The model under review builds one solid part; all positions refer to its coordinate system, in mm. Face numbers are marked on the shaded views. Coordinates: 2 decimals unless noted, no trailing zeros. Write each loop counter-clockwise with the first axis right and the second up, starting at its lowest first coordinate (ties: lowest second). Pieces come first, ordered by that corner, then holes.
1) For P1, Ø5, axis at y = 19.5, z = 2, coming from the +X side; P2, Ø2.5, axis at x = 28.28, y = 28.28, coming from the +Z side; P3, Ø5, axis at y = 20, z = 4.5, coming from the +X side, all flat-tipped, find the tip position at first contact; note any pin that passes through.
2) Add section B-B, the plane y = 14. State the section outline as (x, z) points, then the cut area to 3 significant figures.
3) For line 1 (Y direction, x = 10.5, z = 7); line 2 (Y direction, x = 10, z = 8.25); line 3 (X direction, y = 16.5, z = 6.75), list the stretches that pass through material, from the lowest coordinate up.
4) Add section C-C, the plane z = 2.5. State the section outline as (x, y) points, then the cut area to 3 significant figures.
5) Add section A-A, the plane x = 12.5. State the section outline as (y, z) points.
6) Mouldability with a two-part tool opening along Y and no side actions: class the marked faces 1, 2, 3 and 4 as released by +Y, released by -Y, zero draft, split by the parting line, or undercut.
7) Add section D-D, the plane x = 32. State the section outline as (y, z) points.
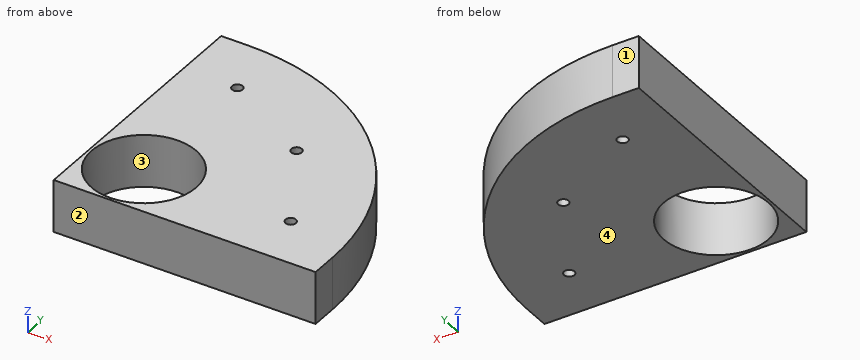
from build123d import *

# Parameters (mm, degrees)
F0_W     = 50
F0_H     = 50
F1_DEPTH = 10
F3_R     = 45
F2_R     = 10
F5_DEPTH = 10.001
F4_R     = 1
F6_DEPTH = 10.001


with BuildPart() as f1:
    # F0 (on Top) → F1 (new body)
    with BuildSketch(Plane.XY):
        with Locations((25, 25)):
            Rectangle(F0_W, F0_H)
    extrude(amount=F1_DEPTH)

    # F3
    f3_edges = [f1.edges().sort_by_distance(p)[0] for p in [
        (50, 50, 5),
    ]]
    fillet(f3_edges, radius=F3_R)

    # F2 (on face) → F5 (cut, through all)
    with BuildSketch(Plane(origin=(0, 0, 0), x_dir=(1, 0, 0), z_dir=(0, 0, -1))):
        with Locations((10.5, -10.5)):
            Circle(F2_R)
    extrude(amount=-F5_DEPTH, mode=Mode.SUBTRACT)

    # F4 (on face) → F6 (cut, through all)
    with BuildSketch(Plane(origin=(0, 0, 0), x_dir=(1, 0, 0), z_dir=(0, 0, -1))):
        with Locations((10.352762, -38.637033)):
            Circle(F4_R)
        with Locations((28.284271, -28.284271)):
            Circle(F4_R)
        with Locations((38.637033, -10.352762)):
            Circle(F4_R)
    extrude(amount=-F6_DEPTH, mode=Mode.SUBTRACT)


solid = f1.part
Geometry results:
1. P1: stops at x = 48.37
1. P2: stops at z = 10
1. P3: stops at x = 48.23
2. outline: (0, 0) - (1.13, 0) - (1.13, 10) - (0, 10) - close; (19.87, 0) - (49.09, 0) - (49.09, 10) - (19.87, 10) - close
2. area: 304 mm2
3. line 1: y = 0 to 0.5, 20.5 to 37.65, 39.63 to 49.66
3. line 2: y = 0 to 0.51, 20.49 to 37.7, 39.57 to 49.72
3. line 3: x = 0 to 2.5, 18.5 to 48.51
4. outline: (0, 0) - (50, 0) - (50, 5) arc R45 ccw to (5, 50) - (0, 50) - close; hole circle Ø20 at (10.5, 10.5); hole circle Ø2 at (10.35, 38.64); hole circle Ø2 at (28.28, 28.28); hole circle Ø2 at (38.64, 10.35)
4. area: 1,740 mm2
5. outline: (0, 0) - (0.7, 0) - (0.7, 10) - (0, 10) - close; (20.3, 0) - (49.37, 0) - (49.37, 10) - (20.3, 10) - close
6. face 1: released by +Y
6. face 2: released by -Y
6. face 3: undercut
6. face 4: zero draft
7. outline: (0, 0) - (41, 0) - (41, 10) - (0, 10) - close
